```python
from build123d import *


with BuildPart() as part:
    # Sweep1: sweep along a path in Sketch1
    with BuildLine(Plane.XY) as sweep1_path:
        Line((0, 0), (-60, 0))
        ThreePointArc((-60, 0), (-63.535533906, -1.464466094), (-65, -5))
        Line((-65, -5), (-65, -20))
    # Sketch2 → Sweep1 (sweep)
    with BuildSketch(Plane.ZY):
        Polygon((1.720776661, -3.006480947), (3.464077206, -0.013004171), (1.743300546, 2.993476776), (-1.720776661, 3.006480947), (-3.464077206, 0.013004171), (-1.743300546, -2.993476776), align=None)
    sweep(path=sweep1_path.line)


solid = part.part
```
CAD build for the part. Positions are in the model's coordinates, mm. A direction names the side the tool comes from. Round coordinates to 2 decimals unless told otherwise and drop trailing zeros. Order: outer loops, then holes, each group sorted by start corner. A loop starts at its lowest first (then second) coordinate and runs counter-clockwise, first axis right, second up. Notation, with made-up numbers: (53.5, -10) - (105.5, -10) arc R10 cw to (105.5, 1) - close; hole circle Ø6 at (0.5, 80.5). An arc over 180 degrees is marked (long way). Answer in a Markdown table with one row per item. Add a question column.
(1) Drop flat-ended pins along their axis: pin 1 Ø4 at (y, z) = (-16.5, -1) entering from +X; pin 2 Ø1 at (y, z) = (-4, 2.5) entering from -X. Give the stop position or say it passes through.
(2) Probe L1, parallel to X at y = -17.25, z = 1.5; L2, parallel to Y at x = -48, z = -1.5; L3, parallel to Z at x = -35, y = -1. List the from-to ranges inside material, lowest first. Write a range as [from, to].
(3) Band-saw the part on B-B on x = -37. List the corners of the cut face in (y, z).
(4) Band-saw the part on A-A on y = -10.75. List the corners of the cut face in (x, z), and give its area (3 significant figures).
(5) 3-axis set-ups, long thin cutter, end or side, ignore diameter. For faces 1 (the face through (-63.5, -12.6, 2.6)), 2 (the face through (-63.5, -12.6, -2.6)): which of +Z, -Z, +X, -X, +Y, -Y reach the whole face in a straight line?
(6) Band-saw the part on C-C on z = 0.75. List the corners of the cut face in (x, y), and give its area (3 significant figures).
Data:
| question | item | result |
|---|---|---|
| 1 | pin 1 | stops at x = -62 |
| 1 | pin 2 | stops at x = -67.48 |
| 2 | L1 | x = [-67.99, -61.99] |
| 2 | L2 | y = [-2.99, 3.01] |
| 2 | L3 | z = [-2.88, 2.89] |
| 3 | outline | (-3.01, 1.72) - (-2.99, -1.74) - (0.01, -3.46) - (3.01, -1.72) - (2.99, 1.74) - (-0.01, 3.46) - close |
| 4 | outline | (-68.01, -1.72) - (-65.01, -3.46) - (-62.01, -1.74) - (-61.99, 1.72) - (-64.99, 3.46) - (-67.99, 1.74) - close |
| 4 | area | 31.2 mm^2 |
| 5 | face 1 | +Z, +X, -Y |
| 5 | face 2 | -Z, +X, -Y |
| 6 | outline | (-68, -20) - (-62, -20) - (-62, -5) arc R2 cw to (-60, -3) - (0, -3) - (0, 3) - (-60, 3) arc R8 ccw to (-68, -5) - close |
| 6 | area | 497 mm^2 |
